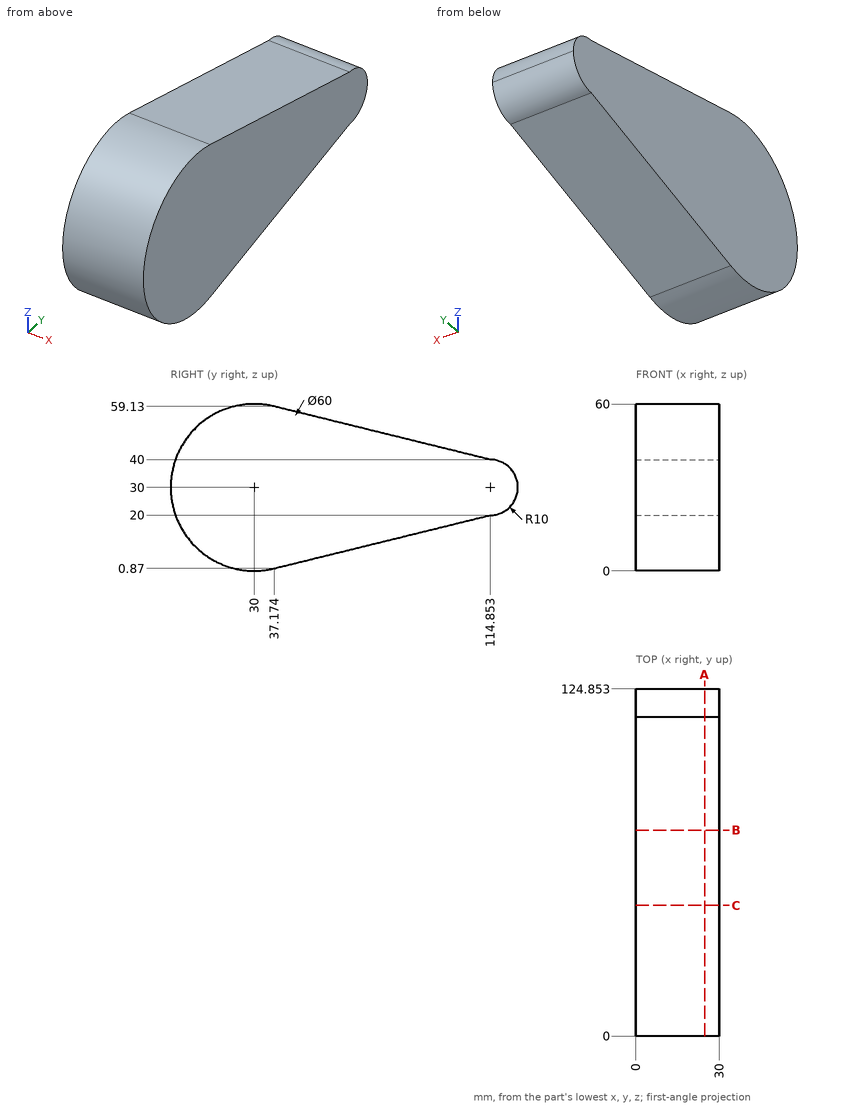
Check sheet for the drawn part. Datum: minimum x, y, z corner. Units: mm. Coordinates: 2 decimals unless noted, no trailing zeros. Write each loop counter-clockwise with the first axis right and the second up, starting at its lowest first coordinate (ties: lowest second). Pieces come first, ordered by that corner, then holes. Notation, with made-up numbers: (-26, 28.25) - (-1, 28.25) arc R27 ccw to (-1, 60.25) - close; hole circle Ø11 at (19.5, 3.5). An arc over 180 degrees is marked (long way). Answer as a JSON object with one key per item and string values.
(1) Gauge pin test, flat ends, axial feed: pin 1 Ø4 at (x, y) = (11, 40) entering from -Z; pin 2 Ø8 at (x, y) = (8.5, 91.5) entering from +Z; pin 3 Ø1 at (x, z) = (5.5, 48) entering from -Y. Record the tip position at first contact, or that the pin passes through.
Report:
{"pin 1": "z = 1.07", "pin 2": "z = 46.74", "pin 3": "y = 5.63"}
(2) Cross-section at C-C on y = 47. Record the cut outline in (x, z), plus the area to 3 significant figures.
Report:
{"outline": "(0, 3.29) - (30, 3.29) - (30, 56.71) - (0, 56.71) - close", "area": "1,600 mm^2"}
(3) Thickness scan on line 1 along Y through (x, z) = (11.5, 21.5); line 2 along Z through (x, y) = (16, 55.5); line 3 along Z through (x, y) = (21.25, 29). Record the ranges inside material, lowest first.
Report:
{"line 1": "1.23 to 120.12", "line 2": "5.38 to 54.62", "line 3": "0.02 to 59.98"}
(4) Cross-section at B-B on y = 74. Record the cut outline in (x, z).
Report:
{"outline": "(0, 9.94) - (30, 9.94) - (30, 50.06) - (0, 50.06) - close"}
(5) Cross-section at A-A on x = 24.75. Record the cut outline in (y, z).
Report:
{"outline": "(37.17, 0.87) - (114.85, 20) arc R10 ccw to (114.85, 40) - (37.17, 59.13) arc R30 ccw (long way) to start"}
